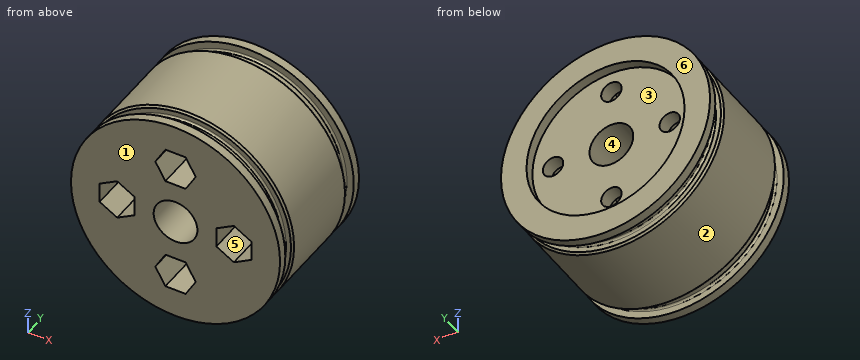
from build123d import *

# Parameters (mm, degrees)
SKETCH1_R           = 21.5
SKETCH1_R_2         = 4.5
SKETCH1_R_3         = 2.1
BOSS_EXTRUDE1_DEPTH = 27
CUT_EXTRUDE1_DEPTH  = 22
SKETCH3_R           = 16.25
CUT_EXTRUDE2_DEPTH  = 2
SKETCH6_R           = 21.5
SKETCH6_R_2         = 19.7
CUT_EXTRUDE3_DEPTH  = 2.6
CUT_EXTRUDE4_START  = -2.6
SKETCH7_R           = 21.5
SKETCH7_R_2         = 19.7
CUT_EXTRUDE4_DEPTH  = 2.6
FILLET1_R           = 0.4
CHAMFER1_SIZE       = 0.4


with BuildPart() as part:
    # Sketch1 → Boss-Extrude1 (new body)
    with BuildSketch(Plane(origin=(0, 0, 0), x_dir=(1, 0, 0), z_dir=(0, 1, 0))):
        with Locations(Location((0, 0, 0), (0, 0, 270))):
            Circle(SKETCH1_R)
        with Locations(Location((0, 0, 0), (0, 0, 270))):
            Circle(SKETCH1_R_2, mode=Mode.SUBTRACT)
        with Locations(Location((0, 12, 0), (0, 0, 270))):
            Circle(SKETCH1_R_3, mode=Mode.SUBTRACT)
        with Locations(Location((12, 0, 0), (0, 0, 270))):
            Circle(SKETCH1_R_3, mode=Mode.SUBTRACT)
        with Locations(Location((0, -12, 0), (0, 0, 270))):
            Circle(SKETCH1_R_3, mode=Mode.SUBTRACT)
        with Locations(Location((-12, 0, 0), (0, 0, 270))):
            Circle(SKETCH1_R_3, mode=Mode.SUBTRACT)
    extrude(amount=BOSS_EXTRUDE1_DEPTH)

    # Sketch2 → Cut-Extrude1 (cut)
    with BuildSketch(Plane.XZ):
        Polygon((12, -4.156921938), (15.6, -2.078460969), (15.6, 2.078460969), (12, 4.156921938), (8.4, 2.078460969), (8.4, -2.078460969), align=None)
        Polygon((4.156921938, 12), (2.078460969, 15.6), (-2.078460969, 15.6), (-4.156921938, 12), (-2.078460969, 8.4), (2.078460969, 8.4), align=None)
        Polygon((-4.156921938, -12), (-2.078460969, -15.6), (2.078460969, -15.6), (4.156921938, -12), (2.078460969, -8.4), (-2.078460969, -8.4), align=None)
        Polygon((-12, 4.156921938), (-15.6, 2.078460969), (-15.6, -2.078460969), (-12, -4.156921938), (-8.4, -2.078460969), (-8.4, 2.078460969), align=None)
    extrude(amount=-CUT_EXTRUDE1_DEPTH, mode=Mode.SUBTRACT)

    # Sketch3 → Cut-Extrude2 (cut)
    with BuildSketch(Plane(origin=(0, 27, 0), x_dir=(1, 0, 0), z_dir=(0, 1, 0))):
        with Locations(Location((0, 0, 0), (0, 0, 270))):
            Circle(SKETCH3_R)
    extrude(amount=-CUT_EXTRUDE2_DEPTH, mode=Mode.SUBTRACT)

    # Sketch6 → Cut-Extrude3 (cut)
    with BuildSketch(Plane(origin=(0, 1.8, 0), x_dir=(-1, 0, 0), z_dir=(0, -1, 0))):
        with Locations(Location((0, 0, 0), (0, 0, 90))):
            Circle(SKETCH6_R)
        with Locations(Location((0, 0, 0), (0, 0, 90))):
            Circle(SKETCH6_R_2, mode=Mode.SUBTRACT)
    extrude(amount=-CUT_EXTRUDE3_DEPTH, mode=Mode.SUBTRACT)

    # Sketch7 → Cut-Extrude4 (cut)
    with BuildSketch(Plane(origin=(0, 25.2, 0), x_dir=(1, 0, 0), z_dir=(0, 1, 0)).offset(CUT_EXTRUDE4_START)):
        with Locations(Location((0, 0, 0), (0, 0, 90))):
            Circle(SKETCH7_R)
        with Locations(Location((0, 0, 0), (0, 0, 90))):
            Circle(SKETCH7_R_2, mode=Mode.SUBTRACT)
    extrude(amount=CUT_EXTRUDE4_DEPTH, mode=Mode.SUBTRACT)

    # Fillet1
    fillet1_edges = [part.edges().sort_by_distance(p)[0] for p in [
        (0, 4.4, 19.7),
        (0, 1.8, 19.7),
        (0, 22.6, 19.7),
        (0, 25.2, 19.7),
    ]]
    fillet(fillet1_edges, radius=FILLET1_R)

    # Chamfer1
    chamfer1_edges = [part.edges().sort_by_distance(p)[0] for p in [
        (0, 4.4, -21.5),
        (0, 22.6, -21.5),
    ]]
    chamfer(chamfer1_edges, length=CHAMFER1_SIZE)


solid = part.part
Can you work these out from the model? Positions are in its coordinate system, mm. Face numbers are marked on the shaded views. A direction names the side the tool comes from. Round coordinates to 2 decimals unless told otherwise and drop trailing zeros. Loops run counter-clockwise (first coordinate to the right, second up) from the corner with the lowest first, then second, coordinate; pieces in that order, holes last. Notation, with made-up numbers: (-37, 43.5) - (-27, 43.5) arc R26 ccw to (-27, 78.5) - close; hole circle Ø10 at (-8.5, 3.25). An arc over 180 degrees is marked (long way). Use CSV: the item, a comma, the result in double quotes. Start each with the question number.
1) For the marked faces 5 and 6, which set-ups out of +Z, -Z, +X, -X, +Y, -Y let a thin tool reach every point of the face, with its end or its side?
2) If we section it at A-A on y = 3: Write out the boundary of the cut face in (x, z), plus the area to 3 significant figures.
3) We'd pull the mould along X, two halves only. Please class the marked faces 1, 2, 3 and 4: released by +X, released by -X, zero draft, split by the parting line, or undercut.
4) If we section it at D-D on y = 16.5: Write out the boundary of the cut face in (x, z), plus the area to 3 significant figures.
5) If we section it at B-B on x = 0: Count the separate pieces of the cut face and the enclosed holes in it, plus the area to 3 significant figures.
6) For pin 1 Ø12 at (x, y) = (-12, 13) entering from -Z; pin 2 Ø6 at (y, z) = (12, -9.5) entering from -X; pin 3 Ø4.5 at (y, z) = (12, 0.5) entering from +X, each with a flat end and sliding along its axis, tell me the tip position at first contact or that it passes through.
7) Please list where these lines run through material, in increasing order: probe 1 along Y at (x, z) = (11, -17); probe 2 along Z at (x, y) = (-4, 21.75); probe 3 along Z at (x, y) = (3, 5.5). Write a range as [from, to].
Geometry results:
1,face 5,"-Y"
1,face 6,"+Z, -Z, +X, -X, +Y"
2,outline,"circle Ø39.4 at (0, 0); hole (-15.6, -2.08) - (-12, -4.16) - (-8.4, -2.08) - (-8.4, 2.08) - (-12, 4.16) - (-15.6, 2.08) - close; hole circle Ø9 at (0, 0); hole (-4.16, -12) - (-2.08, -15.6) - (2.08, -15.6) - (4.16, -12) - (2.08, -8.4) - (-2.08, -8.4) - close; hole (-4.16, 12) - (-2.08, 8.4) - (2.08, 8.4) - (4.16, 12) - (2.08, 15.6) - (-2.08, 15.6) - close; hole (8.4, -2.08) - (12, -4.16) - (15.6, -2.08) - (15.6, 2.08) - (12, 4.16) - (8.4, 2.08) - close"
2,area,"976 mm2"
3,face 1,"zero draft"
3,face 2,"split by the parting line"
3,face 3,"undercut"
3,face 4,"undercut"
4,outline,"circle Ø43 at (0, 0); hole (-15.6, -2.08) - (-12, -4.16) - (-8.4, -2.08) - (-8.4, 2.08) - (-12, 4.16) - (-15.6, 2.08) - close; hole circle Ø9 at (0, 0); hole (-4.16, -12) - (-2.08, -15.6) - (2.08, -15.6) - (4.16, -12) - (2.08, -8.4) - (-2.08, -8.4) - close; hole (-4.16, 12) - (-2.08, 8.4) - (2.08, 8.4) - (4.16, 12) - (2.08, 15.6) - (-2.08, 15.6) - close; hole (8.4, -2.08) - (12, -4.16) - (15.6, -2.08) - (15.6, 2.08) - (12, 4.16) - (8.4, 2.08) - close"
4,area,"1,210 mm2"
5,separate pieces,"4"
5,enclosed holes,"0"
5,area,"510 mm2"
6,pin 1,"stops at z = -20.65"
6,pin 2,"stops at x = -20.49"
6,pin 3,"stops at x = 21.5"
7,probe 1,"y = [0, 1.8], [4.4, 22.6], [25.2, 27]"
7,probe 2,"z = [-21.12, -12.27], [-11.73, -2.06], [2.06, 11.73], [12.27, 21.12]"
7,probe 3,"z = [-21.29, -14], [-10, -3.35], [3.35, 10], [14, 21.29]"
